The listing builds one solid part. Answer for the finished solid, in the listing's coordinates (mm). Face numbers are marked on the shaded views. Round coordinates to 2 decimals unless told otherwise and drop trailing zeros. Order: outer loops, then holes, each group sorted by start corner. A loop starts at its lowest first (then second) coordinate and runs counter-clockwise, first axis right, second up. Notation, with made-up numbers: (40.25, 52.5) - (66.25, 52.5) arc R23 ccw to (66.25, 88.5) - close; hole circle Ø8 at (-28.5, 31). An arc over 180 degrees is marked (long way). Use CSV: the item, a comma, the result in double quotes. Start each with the question number.
Item 1: Find section A-A, the plane y = -25.4. Give the vertices of the cut face in (x, z) (3 decimals), plus the area to 3 significant figures.
Item 2: Find section B-B, the plane x = 44. Give the vertices of the cut face in (y, z) (3 decimals).
Item 3: Find section C-C, the plane z = 25.4. Give the vertices of the cut face in (x, y) (3 decimals), plus the area to 3 significant figures.
Item 4: Straight lines are drawn through the part: line 1 along X through (y, z) = (-25.4, 11.5); line 2 along Y through (x, z) = (31, 41); line 3 along Z through (x, y) = (8.75, -25.4). For each, find the intervals that lie inside material, in ascending order. Write a range as [from, to].
Item 5: Find section D-D, the plane y = -14. Count the separate pieces of the cut face and the enclosed holes in it, plus the area to 3 significant figures.
Item 6: Determine the mould class of the marked faces 1, 2, 3 and 4 for opening direction Y: +Y half, -Y half, draft (parallel to the pull), parting line (faces both ways), or undercut.
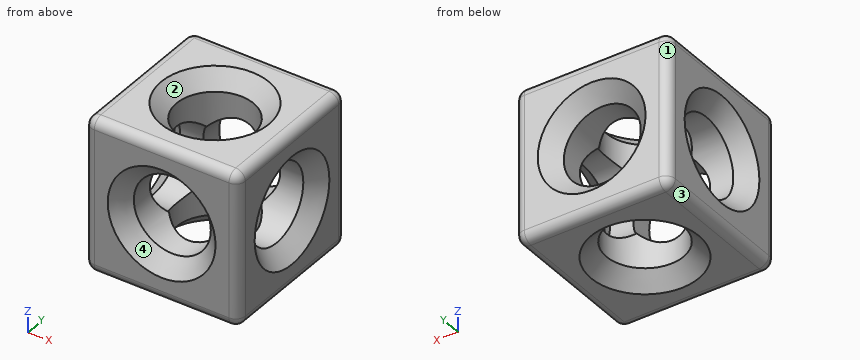
```python
from build123d import *

# Parameters (mm, degrees)
F0_W     = 50.8113652468
F0_H     = 50.8
F1_DEPTH = 50.8
F2_R     = 12.7
F3_DEPTH = 50.8
F4_R     = 12.7
F5_DEPTH = 50.8
F6_DEPTH = 50.8
F7_R     = 12.7
F8_DEPTH = 50.8
F9_R     = 3.175
F10_SIZE = 5.08


with BuildPart() as f1:
    # F0 (on Front) → F1 (new body)
    with BuildSketch(Plane.XZ):
        with Locations((25.4056826234, 25.4)):
            Rectangle(F0_W, F0_H)
    extrude(amount=F1_DEPTH)

    # F2 (on face) → F3 (cut)
    with BuildSketch(Plane.XZ.offset(50.8)):
        with Locations((25.4056826234, 25.4)):
            Circle(F2_R)
    extrude(amount=-F3_DEPTH, mode=Mode.SUBTRACT)

    # F4 (on face) → F5 (cut)
    with BuildSketch(Plane.YZ.offset(50.8113652468)):
        with Locations((-25.4, 25.4)):
            Circle(F4_R)
    extrude(amount=-F5_DEPTH, mode=Mode.SUBTRACT)

    # F6 (cut): a face of the model
    f6_faces = [f1.faces().sort_by_distance(p)[0] for p in [
        (0.0113652468, -25.4, 25.4),
    ]]
    extrude(f6_faces, amount=-F6_DEPTH, mode=Mode.SUBTRACT)

    # F7 (on face) → F8 (cut)
    with BuildSketch(Plane.XY.offset(50.8)):
        with Locations((25.4056826234, -25.4)):
            Circle(F7_R)
    extrude(amount=-F8_DEPTH, mode=Mode.SUBTRACT)

    # F9
    f9_edges = [f1.edges().sort_by_distance(p)[0] for p in [
        (50.811365, -25.4, 50.8),
        (25.405683, -50.8, 50.8),
        (0, -25.4, 50.8),
        (25.405683, 0, 50.8),
        (50.811365, -50.8, 25.4),
        (50.811365, 0, 25.4),
        (50.811365, -25.4, 0),
        (25.405683, -50.8, 0),
        (0, -50.8, 25.4),
        (0, 0, 25.4),
        (25.405683, 0, 0),
        (0, -25.4, 0),
    ]]
    fillet(f9_edges, radius=F9_R)

    # F10
    f10_edges = [f1.edges().sort_by_distance(p)[0] for p in [
        (12.705683, -50.8, 25.4),
        (12.705683, -25.4, 0),
        (0, -25.4, 47.625),
        (0, -3.175, 25.4),
        (0, -47.625, 25.4),
        (0, -25.4, 3.175),
        (0, -38.1, 25.4),
        (12.705683, 0, 25.4),
        (12.705683, -25.4, 50.8),
        (50.811365, -38.1, 25.4),
    ]]
    chamfer(f10_edges, length=F10_SIZE)


solid = f1.part
```
Worked out:
1,outline,"(0, 3.175) arc R3.175 ccw to (3.175, 0) - (7.626, 0) - (12.706, 5.08) - (12.706, 12.7) - (5.08, 12.7) - (0, 7.62) - close; (0, 43.18) - (5.08, 38.1) - (12.706, 38.1) - (12.706, 45.72) - (7.626, 50.8) - (3.175, 50.8) arc R3.175 ccw to (0, 47.625) - close; (38.106, 5.08) - (43.186, 0) - (47.636, 0) arc R3.175 ccw to (50.811, 3.175) - (50.811, 7.62) - (45.731, 12.7) - (38.106, 12.7) - close; (38.106, 38.1) - (45.731, 38.1) - (50.811, 43.18) - (50.811, 47.625) arc R3.175 ccw to (47.636, 50.8) - (43.186, 50.8) - (38.106, 45.72) - close"
1,area,"534 mm²"
2,outline,"(-50.8, 3.175) arc R3.175 ccw to (-47.625, 0) - (-3.175, 0) arc R3.175 ccw to (0, 3.175) - (0, 47.625) arc R3.175 ccw to (-3.175, 50.8) - (-47.625, 50.8) arc R3.175 ccw to (-50.8, 47.625) - close; hole circle Ø25.4 at (-25.4, 25.4)"
3,outline,"(0, -47.625) arc R3.175 ccw to (3.175, -50.8) - (7.626, -50.8) - (12.706, -45.72) - (12.706, -38.1) - (5.08, -38.1) - (0, -43.18) - close; (0, -7.62) - (5.08, -12.7) - (12.706, -12.7) - (12.706, -5.08) - (7.626, 0) - (3.175, 0) arc R3.175 ccw to (0, -3.175) - close; (38.106, -45.72) - (43.186, -50.8) - (47.636, -50.8) arc R3.175 ccw to (50.811, -47.625) - (50.811, -43.18) - (45.731, -38.1) - (38.106, -38.1) - close; (38.106, -12.7) - (45.731, -12.7) - (50.811, -7.62) - (50.811, -3.175) arc R3.175 ccw to (47.636, 0) - (43.186, 0) - (38.106, -5.08) - close"
3,area,"534 mm²"
4,line 1,"x = [3.88, 12.71], [38.11, 46.93]"
4,line 2,"y = [-49.59, -36.8], [-14, -1.21]"
4,line 3,"z = [1.12, 12.7], [38.1, 49.68]"
5,separate pieces,"4"
5,enclosed holes,"0"
5,area,"1,300 mm²"
6,face 1,"+Y half"
6,face 2,"undercut"
6,face 3,"draft"
6,face 4,"-Y half"
